Design review of the part built by this model. Coordinates are the model's own, in mm. Face numbers are marked on the shaded views. Give positions to 0.01 mm unless a question says otherwise; leave off trailing zeros. Order: outer loops, then holes, each group sorted by start corner. A loop starts at its lowest first (then second) coordinate and runs counter-clockwise, first axis right, second up. Notation, with made-up numbers: M 70.25,43.25 L 108.25,43.25 A18 cw 108.25,70.25 Z; hole C 52,-21.75 d9. An arc over 180 degrees is marked long. Put each result on its own line as item: value. Start each with the question number.
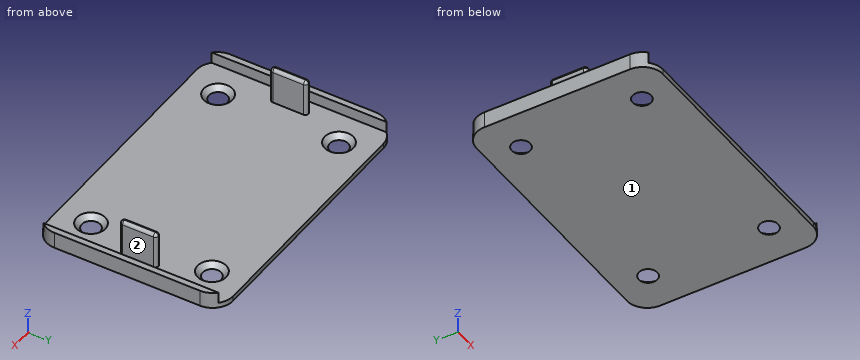
from build123d import *

# Parameters (mm, degrees)
F0_W     = 65.5
F0_H     = 45.5
F0_R     = 1.5
F0_W_2   = 1.5
F0_H_2   = 9
F1_DEPTH = 1.25
F2_DEPTH = 10
F3_DEPTH = 4
F5_R     = 0.74999
F6_R     = 0.74999
F7_R     = 5


# Not quite as in the source:
# - a fillet or chamfer that OpenCascade refuses, or shapes differently, is made with other operations: its cross-section is extruded or revolved along the edge and cut away or added
# - a fillet or chamfer is up to 0.001 mm smaller than in the source, because OpenCascade refuses the exact size


with BuildPart() as f1:
    # F0 (on Top) → F1 (new body)
    with BuildSketch(Plane.XY):
        Rectangle(F0_W, F0_H)
        with Locations((-24.75, -14.75)):
            Circle(F0_R, mode=Mode.SUBTRACT)
        with Locations((24.75, -14.75)):
            Circle(F0_R, mode=Mode.SUBTRACT)
        with Locations((-29.25, 0)):
            Rectangle(F0_W_2, F0_H_2, mode=Mode.SUBTRACT)
        with Locations((-24.75, 14.75)):
            Circle(F0_R, mode=Mode.SUBTRACT)
        with Locations((29.25, 0)):
            Rectangle(F0_W_2, F0_H_2, mode=Mode.SUBTRACT)
        with Locations((24.75, 14.75)):
            Circle(F0_R, mode=Mode.SUBTRACT)
    extrude(amount=F1_DEPTH)

    # F0 (on Top) → F2 (join)
    with BuildSketch(Plane.XY):
        with Locations((-29.25, 0)):
            Rectangle(F0_W_2, F0_H_2)
        with Locations((29.25, 0)):
            Rectangle(F0_W_2, F0_H_2)
    extrude(amount=F2_DEPTH)

    # F0 (on Top) → F3 (join)
    with BuildSketch(Plane.XY):
        with Locations((-33.5, 0)):
            Rectangle(F0_W_2, F0_H)
        with Locations((33.5, 0)):
            Rectangle(F0_W_2, F0_H)
    extrude(amount=F3_DEPTH)

    # F4: chamfer of 2 on 4 edges, made by hand

    # F4_s1 → F4_t2 (revolve, cut)
    with BuildSketch(Plane.XZ.offset(-14.75)):
        Polygon((-21.25, 1.25), (-23.25, -0.75), (-23.25, 1.25), align=None)
    revolve(axis=Axis((-24.75, 14.75, 1.25), (0, 0, 1)), mode=Mode.SUBTRACT)

    # F4_s3 → F4_t4 (revolve, cut)
    with BuildSketch(Plane.XZ.offset(14.75)):
        Polygon((-21.25, 1.25), (-23.25, -0.75), (-23.25, 1.25), align=None)
    revolve(axis=Axis((-24.75, -14.75, 1.25), (0, 0, 1)), mode=Mode.SUBTRACT)

    # F4_s5 → F4_t6 (revolve, cut)
    with BuildSketch(Plane.XZ.offset(-14.75)):
        Polygon((28.25, 1.25), (26.25, -0.75), (26.25, 1.25), align=None)
    revolve(axis=Axis((24.75, 14.75, 1.25), (0, 0, 1)), mode=Mode.SUBTRACT)

    # F4_s7 → F4_t8 (revolve, cut)
    with BuildSketch(Plane.XZ.offset(14.75)):
        Polygon((28.25, 1.25), (26.25, -0.75), (26.25, 1.25), align=None)
    revolve(axis=Axis((24.75, -14.75, 1.25), (0, 0, 1)), mode=Mode.SUBTRACT)

    # F5 (radius 0.75 in the source; OpenCascade refuses exactly that, so slightly less here)
    f5_edges = [f1.edges().sort_by_distance(p)[0] for p in [
        (-30, 4.5, 5.625),
        (30, 4.5, 5.625),
        (28.5, 4.5, 5.625),
        (-30, -4.5, 5.625),
        (-28.5, -4.5, 5.625),
        (28.5, -4.5, 5.625),
        (30, -4.5, 5.625),
        (-28.5, 4.5, 5.625),
    ]]
    fillet(f5_edges, radius=F5_R)

    # F6 (radius 0.75 in the source; OpenCascade refuses exactly that, so slightly less here)
    f6_edges = [f1.edges().sort_by_distance(p)[0] for p in [
        (-29.25, -4.5, 10),
        (-29.780333, -4.280333, 10),
        (-28.719667, -4.280333, 10),
        (-30, 0, 10),
        (-28.5, 0, 10),
        (-29.780333, 4.280333, 10),
        (-28.719667, 4.280333, 10),
        (-29.25, 4.5, 10),
        (29.25, -4.5, 10),
        (28.719667, -4.280333, 10),
        (29.780333, -4.280333, 10),
        (28.5, 0, 10),
        (30, 0, 10),
        (28.719667, 4.280333, 10),
        (29.780333, 4.280333, 10),
        (29.25, 4.5, 10),
    ]]
    fillet(f6_edges, radius=F6_R)

    # F7
    f7_edges = [f1.edges().sort_by_distance(p)[0] for p in [
        (-34.25, -22.75, 2),
        (34.25, -22.75, 2),
        (34.25, 22.75, 2),
        (-34.25, 22.75, 2),
    ]]
    fillet(f7_edges, radius=F7_R)


solid = f1.part
1. Consider section D-D on x = -24.75. Give the boundary of the cut face in (y, z).
2. The part is to be moulded in two halves that separate along X. For the marked faces 1 and 2, say which applies: +X half, -X half, draft (parallel to the pull), parting line (faces both ways), or undercut.
3. Consider section B-B on y = -14.75. Give the boundary of the cut face in (x, z), then the cut area to 3 significant figures.
4. Insertion check: pin 1 (0.8 mm diameter, centred on x = -33.5, y = -6, fed in from +Z); pin 2 (13.5 mm diameter, centred on x = -9, y = 7, fed in from +Z); pin 3 (2.5 mm diameter, centred on y = 2, z = 5.5, fed in from +X). Each pin has a flat end and moves straight along its axis. Give the tip position at first contact, or say it passes through.
5. Consider section A-A on z = 2.25. Give the number of separate pieces and of enclosed holes in the cut face, then the cut area to 3 significant figures.
6. To check wall thickness, follow probe 1 along X at (y, z) = (3, 3); probe 2 along X at (y, z) = (-17, 3.5); probe 3 along Z at (x, y) = (30.5, -10). State the ranges of each line that lie inside material, in increasing order.
Returned:
1. outline: M -22.75,0 L -17,0 L -18.25,1.25 L -22.75,1.25 Z; M -12.5,0 L 12.5,0 L 11.25,1.25 L -11.25,1.25 Z; M 17,0 L 22.75,0 L 22.75,1.25 L 18.25,1.25 Z
2. face 1: draft
2. face 2: undercut
3. outline: M -34.25,0 L -27,0 L -28.25,1.25 L -32.75,1.25 L -32.75,4 L -34.25,4 Z; M -22.5,0 L 22.5,0 L 21.25,1.25 L -21.25,1.25 Z; M 27,0 L 34.25,0 L 34.25,4 L 32.75,4 L 32.75,1.25 L 28.25,1.25 Z
3. area: 79.5 mm2
4. pin 1: stops at z = 4
4. pin 2: stops at z = 1.25
4. pin 3: stops at x = 30
5. separate pieces: 4
5. enclosed holes: 0
5. area: 147 mm2
6. probe 1: x = -34.25 to -32.75, -30 to -28.5, 28.5 to 30, 32.75 to 34.25
6. probe 2: x = -34.25 to -32.75, 32.75 to 34.25
6. probe 3: z = 0 to 1.25
